Design review of the part shown in the three views and the two pictorial views. Dimensions are in mm from the part's minimum x, y and z. Coordinates: 2 decimals unless noted, no trailing zeros. Order: outer loops, then holes, each group sorted by start corner. A loop starts at its lowest first (then second) coordinate and runs counter-clockwise, first axis right, second up. Notation, with made-up numbers: (30, 61.5) -> (79, 61.5) arc R34 cw to (79, 98.5) -> close; hole circle Ø1 at (9.25, -23). An arc over 180 degrees is marked (long way). Write item = value, one per line. Start each with the question number.
1) Consider section C-C on y = 7.25. Give the boundary of the cut face in (x, z).
2) Wall thickness on probe 1 along X at (y, z) = (7, 6.25); probe 2 along Z at (x, y) = (6.75, 4.75); probe 3 along Z at (x, y) = (9.25, 9.75): over which ranges is each line inside the solid? List them lowest first. Write a range as [from, to].
3) Consider section B-B on x = 7.25. Give the boundary of the cut face in (y, z).
4) Consider section A-A on z = 5.25. Give the boundary of the cut face in (x, y), and give its area (3 significant figures).
5) Consider section D-D on z = 11. Give the boundary of the cut face in (x, y).
6) Insertion check: pin 1 Ø4.5 at (x, z) = (7.5, 7.5) entering from -Y; pin 2 Ø1 at (y, z) = (5, 4.5) entering from +X; pin 3 Ø1.5 at (x, y) = (9.5, 4.5) entering from +Z; pin 4 Ø1 at (y, z) = (2, 6) entering from -X. Each pin has a flat end and moves straight along its axis. Give the tip position at first contact, or say it passes through.
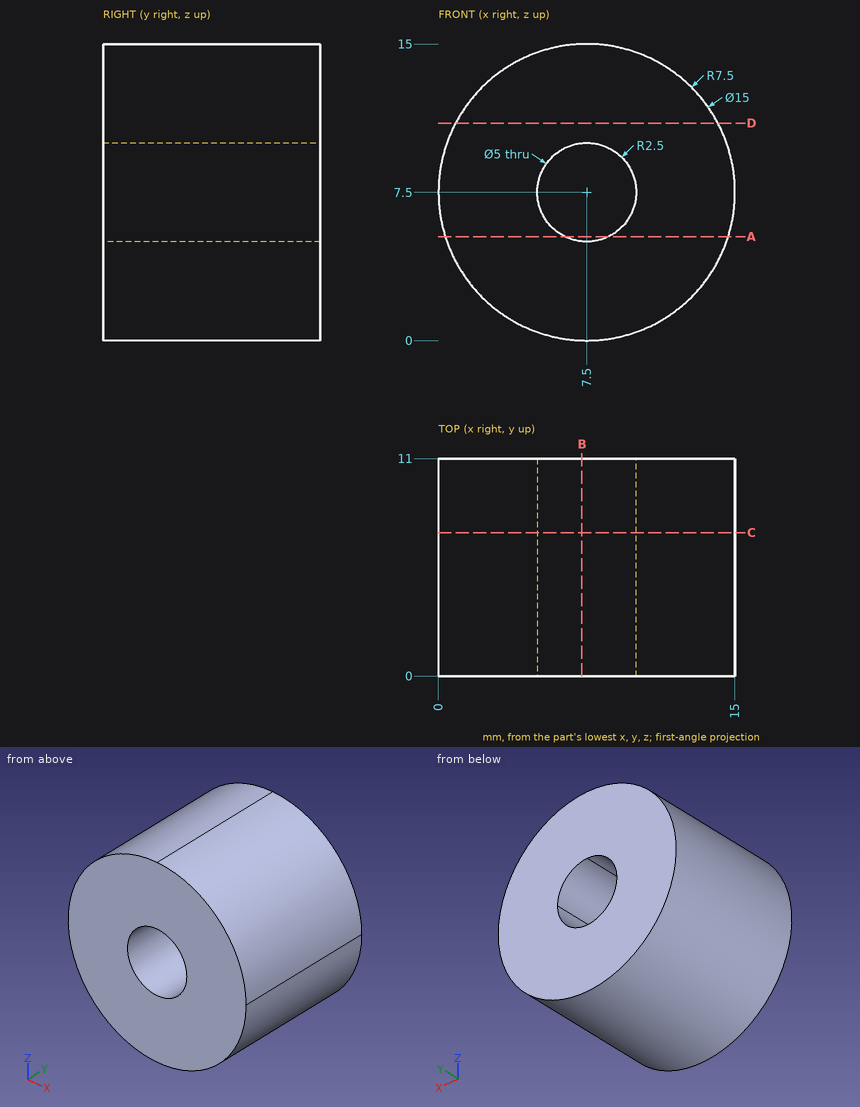
Answer sheet:
q1.outline = circle Ø15 at (7.5, 7.5); hole circle Ø5 at (7.5, 7.5)
q2.probe_1 = [0.1, 5.33], [9.67, 14.9]
q2.probe_2 = [0.04, 5.12], [9.88, 14.96]
q2.probe_3 = [0.21, 5.71], [9.29, 14.79]
q3.outline = (0, 0) -> (11, 0) -> (11, 5.01) -> (0, 5.01) -> close; (0, 9.99) -> (11, 9.99) -> (11, 15) -> (0, 15) -> close
q4.outline = (0.35, 0) -> (6.41, 0) -> (6.41, 11) -> (0.35, 11) -> close; (8.59, 0) -> (14.65, 0) -> (14.65, 11) -> (8.59, 11) -> close
q4.area = 133 mm2
q5.outline = (0.87, 0) -> (14.13, 0) -> (14.13, 11) -> (0.87, 11) -> close
q6.pin_1 = through
q6.pin_2 = 14.57
q6.pin_3 = 14.9
q6.pin_4 = 0.07
